```python
from build123d import *

# Parameters (mm, degrees)
SKETCH_1_W             = 30
SKETCH_1_H             = 13
EXTRUDE_1_DEPTH        = 4
SKETCH_3_R             = 4.7
CUT_EXTRUDE_2_DEPTH    = 10
HOLE_WIZARD_M2_1_D     = 1.6
HOLE_WIZARD_M2_1_DEPTH = 6
HOLE_WIZARD_M2_1_TIP   = 0.480688495
SKETCH_7_W             = 30
SKETCH_7_H             = 7
CUT_EXTRUDE_3_DEPTH    = 10
CHAMFER_1_SIZE         = 3
SKETCH_8_R             = 1.4
CUT_EXTRUDE_4_DEPTH    = 10


with BuildPart() as part:
    # 草图1 → 凸台-拉伸1 (new body)
    with BuildSketch(Plane.XY):
        Rectangle(SKETCH_1_W, SKETCH_1_H)
    extrude(amount=EXTRUDE_1_DEPTH)

    # 草图3 → 切除-拉伸2 (cut)
    with BuildSketch(Plane.XY.offset(4)):
        with Locations((0, 9.854101966)):
            Circle(SKETCH_3_R)
    extrude(amount=-CUT_EXTRUDE_2_DEPTH, mode=Mode.SUBTRACT)

    # M2 螺纹孔1
    with Locations(Plane(origin=(0, -0.645898034, 4), x_dir=(1, 0, 0), z_dir=(0, 0, 1))):
        with Locations((0, 0)):
            Hole(HOLE_WIZARD_M2_1_D / 2, depth=HOLE_WIZARD_M2_1_DEPTH)
            with Locations((0, 0, -(HOLE_WIZARD_M2_1_DEPTH + HOLE_WIZARD_M2_1_TIP / 2))):  # 118° drill point
                Cone(0, HOLE_WIZARD_M2_1_D / 2, HOLE_WIZARD_M2_1_TIP, mode=Mode.SUBTRACT)

    # 草图7 → 切除-拉伸3 (cut)
    with BuildSketch(Plane.XY.offset(4)):
        with Locations((0, -3)):
            Rectangle(SKETCH_7_W, SKETCH_7_H)
    extrude(amount=-CUT_EXTRUDE_3_DEPTH, mode=Mode.SUBTRACT)

    # 倒角1
    chamfer_1_edges = [part.edges().sort_by_distance(p)[0] for p in [
        (-15, 0.5, 2),
        (15, 0.5, 2),
    ]]
    chamfer(chamfer_1_edges, length=CHAMFER_1_SIZE)

    # 草图8 → 切除-拉伸4 (cut)
    with BuildSketch(Plane.XZ.offset(-0.5)):
        with Locations(Location((-10.5, 2, 0), (0, 0, 270))):
            Circle(SKETCH_8_R)
    cut_extrude_4 = extrude(amount=-CUT_EXTRUDE_4_DEPTH, mode=Mode.SUBTRACT)

    # 镜向1: 切除-拉伸4 across plane
    add(cut_extrude_4.mirror(Plane(origin=(0, 0, 0), x_dir=(0, 0, 1), z_dir=(1, 0, 0))), mode=Mode.SUBTRACT)


solid = part.part
```
Design review of the part built by this model. Coordinates are the model's own, in mm. Coordinates: 2 decimals unless noted, no trailing zeros. Loops run counter-clockwise (first coordinate to the right, second up) from the corner with the lowest first, then second, coordinate; pieces in that order, holes last.
Q1. We need section A-A on z = 2. State the section outline as (x, y) points.
Reported:
outline: (-15, 3.5) - (-12, 0.5) - (-11.9, 0.5) - (-11.9, 6.5) - (-15, 6.5) - close; (-9.1, 0.5) - (9.1, 0.5) - (9.1, 6.5) - (3.29, 6.5) arc R4.7 cw to (-3.29, 6.5) - (-9.1, 6.5) - close; (11.9, 0.5) - (12, 0.5) - (15, 3.5) - (15, 6.5) - (11.9, 6.5) - close
Q2. We need section D-D on y = 2.75. State the section outline as (x, z) points.
Reported:
outline: (-14.25, 0) - (14.25, 0) - (14.25, 4) - (-14.25, 4) - close; hole circle Ø2.8 at (-10.5, 2); hole circle Ø2.8 at (10.5, 2)
Q3. The part is to be moulded in two halves that separate along X. For faces 1 (the face through (9, 6.5, 3)), 2 (the face through (-13.5, 2, 2)), 3 (the face through (9.32, 3.46, 1.25)), 4 (the face through (-9.32, 3.46, 1.25)), say which applies: +X half, -X half, draft (parallel to the pull), parting line (faces both ways), or undercut.
Reported:
face 1: draft
face 2: -X half
face 3: undercut
face 4: undercut
Q4. To check wall thickness, follow line 1 (X direction, y = 4.55, z = 2); line 2 (X direction, y = 2, z = 2.2); line 3 (X direction, y = 6.25, z = 1.9). State the ranges of each line that lie inside material, in increasing order.
Reported:
line 1: x = -15 to -11.9, -9.1 to 9.1, 11.9 to 15
line 2: x = -13.5 to -11.89, -9.11 to 9.11, 11.89 to 13.5
line 3: x = -15 to -11.9, -9.1 to -3.02, 3.02 to 9.1, 11.9 to 15
Q5. We need section B-B on x = 10.5. State the section outline as (y, z) points.
Reported:
outline: (0.5, 0) - (6.5, 0) - (6.5, 0.6) - (0.5, 0.6) - close; (0.5, 3.4) - (6.5, 3.4) - (6.5, 4) - (0.5, 4) - close
Q6. We need section C-C on y = 5.75. State the section outline as (x, z) points.
Reported:
outline: (-15, 0) - (-2.29, 0) - (-2.29, 4) - (-15, 4) - close; (2.29, 0) - (15, 0) - (15, 4) - (2.29, 4) - close; hole circle Ø2.8 at (-10.5, 2); hole circle Ø2.8 at (10.5, 2)
